Work out the finished part from the listing and answer in its coordinate system (mm). A direction names the side the tool comes from. Give positions to 0.01 mm unless a question says otherwise; leave off trailing zeros. Loops run counter-clockwise (first coordinate to the right, second up) from the corner with the lowest first, then second, coordinate; pieces in that order, holes last. Notation, with made-up numbers: M -22,-10.5 L 14,-10.5 A20 ccw 14,5.5 Z; hole C 71.5,12 d6. An arc over 180 degrees is marked long. Use a Markdown table: item, result.
```python
from build123d import *

# Parameters (mm, degrees)
PAD_DEPTH       = 37
SKETCH001_W     = 92
SKETCH001_H     = 92
POCKET_DEPTH    = 20
SKETCH002_R     = 11
SKETCH002_R_2   = 5
PAD001_DEPTH    = 2
SKETCH003_R     = 1.5
POCKET001_DEPTH = 5
PAD002_DEPTH    = 24
SKETCH005_W     = 5
SKETCH005_H     = 16
PAD003_DEPTH    = 10


with BuildPart() as part:
    # Sketch → Pad (new body)
    with BuildSketch(Plane.XY):
        Polygon((0, 3.535534), (3.535534, 0), (38.464466, 0), (42, 3.535534), (42, 38.464466), (38.464466, 42), (3.535534, 42), (0, 38.464466), align=None)
    extrude(amount=PAD_DEPTH)

    # Sketch001 (on DatumPlane) → Pocket (cut)
    with BuildSketch(Plane.XY.offset(9)):
        with Locations((21, 21)):
            Rectangle(SKETCH001_W, SKETCH001_H)
        Polygon((34.928932, 42), (42, 34.928932), (42, 7.071068), (34.928932, 0), (7.071068, 0), (0, 7.071068), (0, 34.928932), (7.071068, 42), align=None, mode=Mode.SUBTRACT)
    extrude(amount=POCKET_DEPTH, mode=Mode.SUBTRACT)

    # Sketch002 (on DatumPlane) → Pad001 (join)
    with BuildSketch(Plane.XY.offset(37)):
        with Locations((21, 21)):
            Circle(SKETCH002_R)
        with Locations((21, 21)):
            Circle(SKETCH002_R_2, mode=Mode.SUBTRACT)
    extrude(amount=PAD001_DEPTH)

    # Sketch003 (on DatumPlane) → Pocket001 (cut)
    with BuildSketch(Plane.XY.offset(37)):
        with Locations((5.5, 36.5)):
            Circle(SKETCH003_R)
        with Locations((36.5, 36.5)):
            Circle(SKETCH003_R)
        with Locations((36.5, 5.5)):
            Circle(SKETCH003_R)
        with Locations((5.5, 5.5)):
            Circle(SKETCH003_R)
    extrude(amount=-POCKET001_DEPTH, mode=Mode.SUBTRACT)

    # Sketch004 (on DatumPlane) → Pad002 (join)
    with BuildSketch(Plane.XY.offset(37)):
        with BuildLine():
            ThreePointArc((23, 22.5), (18.5, 21), (23, 19.5))
            Line((23, 19.5), (23, 22.5))
        make_face()
    extrude(amount=PAD002_DEPTH)

    # Sketch005 → Pad003 (join)
    with BuildSketch(Plane.XY):
        with Locations((-2.5, 21)):
            Rectangle(SKETCH005_W, SKETCH005_H)
    extrude(amount=PAD003_DEPTH)


solid = part.part
```
(1) Given P1, Ø5.5, axis at x = -2.5, z = 7.5, coming from the -Y side; P2, Ø3.5, axis at y = 21.5, z = 44, coming from the +X side; P3, Ø1, axis at x = 2, y = 7, coming from the -Z side; P4, Ø2.5, axis at x = -2.5, z = 5, coming from the +Y side, each flat-ended and moving along its own axis, determine where each tip first touches the part or whether it passes through.
Entries:
| item | result |
|---|---|
| P1 | stops at y = 3.29 |
| P2 | stops at x = 23 |
| P3 | stops at z = 0 |
| P4 | stops at y = 29 |
(2) A cutting plane is placed at C-C (x = 19.5). Write down the section's boundary in (y, z), and give its area (3 significant figures).
Entries:
| item | result |
|---|---|
| outline | M 0,0 L 42,0 L 42,37 L 31.9,37 L 31.9,39 L 25.77,39 L 25.77,37 L 23,37 L 23,61 L 19,61 L 19,37 L 16.23,37 L 16.23,39 L 10.1,39 L 10.1,37 L 0,37 Z |
| area | 1,670 mm² |
(3) A cutting plane is placed at B-B (z = 5.5). Write down the section's boundary in (x, y), and give its area (3 significant figures).
Entries:
| item | result |
|---|---|
| outline | M -5,13 L 0,13 L 0,3.54 L 3.54,0 L 38.46,0 L 42,3.54 L 42,38.46 L 38.46,42 L 3.54,42 L 0,38.46 L 0,29 L -5,29 Z |
| area | 1,820 mm² |
(4) A cutting plane is placed at D-D (z = 19). Write down the section's boundary in (x, y).
Entries:
| item | result |
|---|---|
| outline | M 0,7.07 L 7.07,0 L 34.93,0 L 42,7.07 L 42,34.93 L 34.93,42 L 7.07,42 L 0,34.93 Z |
(5) Which of the six approach directions +Z, -Z, +X, -X, +Y, -Y give full straight-line access (tool end or side, diameter ignored) to faces 1 (the flat face through (3, 3, 29)), 2 (the flat face through (39, 39, 9)), 3 (the flat face through (38.514, 3.585, 18.86)), 4 (the cylindrical face through (19.92, 16.12, 37.99))?
Entries:
| item | result |
|---|---|
| face 1 | -X, -Y |
| face 2 | +X, +Y |
| face 3 | +X, -Y |
| face 4 | +Z |
(6) Consider probe 1 along Y at (x, z) = (5, 36); probe 2 along Z at (x, y) = (4.5, 10); probe 3 along X at (y, z) = (32.5, 12). Determine where each line is inside the solid, lowest interval first. Write a range as [from, to].
Entries:
| item | result |
|---|---|
| probe 1 | y = [0, 4.09], [6.91, 35.09], [37.91, 42] |
| probe 2 | z = [0, 37] |
| probe 3 | x = [0, 42] |
(7) The mould has two halves that part along Z. Classify faces 5 (the flat face through (26, 19, 39)), 6 (the flat face through (39, 3, 9)), 7 (the flat face through (40.207, 1.743, 4.437)): released by +Z, released by -Z, zero draft, split by the parting line, or undercut.
Entries:
| item | result |
|---|---|
| face 5 | released by +Z |
| face 6 | undercut |
| face 7 | zero draft |
(8) A cutting plane is placed at A-A (y = 21). Write down the section's boundary in (x, z), and give its area (3 significant figures).
Entries:
| item | result |
|---|---|
| outline | M -5,0 L 42,0 L 42,37 L 32,37 L 32,39 L 26,39 L 26,37 L 23,37 L 23,61 L 18.5,61 L 18.5,37 L 16,37 L 16,39 L 10,39 L 10,37 L 0,37 L 0,10 L -5,10 Z |
| area | 1,740 mm² |
